```python
from build123d import *

# Parameters (mm, degrees)
SKETCH1_R               = 10
SKETCH1_R_2             = 6.1
BOSS_EXTRUDE1_DEPTH     = 20
SKETCH2_R               = 7
SKETCH2_R_2             = 4
BOSS_EXTRUDE2_DEPTH     = 20
CUT_EXTRUDE1_DEPTH      = 31.000000167
CUT_EXTRUDE1_DEPTH_BACK = 31.000000167
SKETCH5_R               = 6.1


# Read off the part's stored shape, not the designer's step: M3 Tapped Hole1
with BuildPart() as part:
    # Sketch1 → Boss-Extrude1 (new, symmetric)
    with BuildSketch(Plane.XY):
        Circle(SKETCH1_R)
        Circle(SKETCH1_R_2, mode=Mode.SUBTRACT)
    extrude(amount=BOSS_EXTRUDE1_DEPTH, both=True)

    # Sketch2 → Boss-Extrude2 (add, symmetric)
    with BuildSketch(Plane(origin=(0, 0, 0), x_dir=(0, 0, -1), z_dir=(1, 0, 0))):
        Circle(SKETCH2_R)
        with Locations(Location((0, 0, 0), (0, 0, 180))):
            Circle(SKETCH2_R_2, mode=Mode.SUBTRACT)
    extrude(amount=BOSS_EXTRUDE2_DEPTH, both=True)

    # M3 Tapped Hole1 outline → M3 Tapped Hole1 (revolve, cut)
    with BuildSketch(Plane(origin=(17, 0, 0), x_dir=(1, 0, 0), z_dir=(0, 0, 1))):
        Polygon((1.525056823, 7.000056823), (0, 7.000056823), (0, 3.799585789), (1.25, 3.799585789), (1.25, 6.725), align=None)
    revolve(axis=Axis((17, 0, 0), (0, 1, 0)), mode=Mode.SUBTRACT)

    # M3 Tapped Hole1 2 outline → M3 Tapped Hole1 2 (revolve, cut)
    with BuildSketch(Plane(origin=(-17, 0, 0), x_dir=(1, 0, 0), z_dir=(0, 0, 1))):
        Polygon((1.525056823, 7.000056823), (0, 7.000056823), (0, 3.799585789), (1.25, 3.799585789), (1.25, 6.725), align=None)
    revolve(axis=Axis((-17, 0, 0), (0, 1, 0)), mode=Mode.SUBTRACT)

    # Sketch5 → Cut-Extrude1 (cut, two sides: drawn at the far end of the back side and taken through both)
    with BuildSketch(Plane.XY.offset(-CUT_EXTRUDE1_DEPTH_BACK)):
        Circle(SKETCH5_R)
    extrude(amount=CUT_EXTRUDE1_DEPTH + CUT_EXTRUDE1_DEPTH_BACK, mode=Mode.SUBTRACT)


solid = part.part
```
Input: part model. Units: mm. Frame: model coordinates. A direction names the side the tool comes from. Give positions to 0.01 mm unless a question says otherwise; leave off trailing zeros. Write each loop counter-clockwise with the first axis right and the second up, starting at its lowest first coordinate (ties: lowest second). Pieces come first, ordered by that corner, then holes. Notation, with made-up numbers: (73, 16.5) - (91, 16.5) arc R20 ccw to (91, 52.5) - close; hole circle Ø5 at (-14, 69.5). An arc over 180 degrees is marked (long way). Write item = value, one per line. Start each with the question number.
1. Section query D-D, the plane z = -6. Output: boundary loops of the cut face in (x, y).
2. Section query B-B, the plane z = 0. Count the separate pieces of the cut face and the enclosed holes in it, then the cut area to 3 significant figures.
3. Mould query, pull axis Z, two halves, no side actions, for faces 1 (the cylindrical face through (10, 0, 0)), 2 (the cylindrical face through (18.155, 5.283, 0.479)), 3 (the flat face through (-20, -3, -3)), 4 (the cylindrical face through (-13.481, -6.834, 1.517)). Classes: released by +Z, released by -Z, zero draft, split by the parting line, or undercut.
4. Access query for faces 5 (the cylindrical face through (-15.845, 5.283, 0.479)), 6 (the cylindrical face through (-2.17, -9.76, 0.28)), 7 (the cylindrical face through (14.507, -3.966, -0.521)), 8 (the cylindrical face through (-14.66, -2.7, -2.95)). Directions: +Z, -Z, +X, -X, +Y, -Y. A direction counts if a zero-diameter tool reaches every point of the face in a straight line with its end or side. Return the directions, or none.
5. Ray query, L1, parallel to X at y = 0, z = 12.75; L2, parallel to Y at x = -2, z = 10. Return the intervals inside material, ascending.
6. Section query A-A, the plane x = 0. Output: boundary loops of the cut face in (y, z).
7. Section query C-C, the plane y = 0. Output: boundary loops of the cut face in (x, z), then the cut area to 3 significant figures.
8. First-contact query: pin 1 Ø1.5 at (x, z) = (-4, -14) entering from -Y; pin 2 Ø8 at (y, z) = (0.5, 9.5) entering from -X; pin 3 Ø12 at (x, z) = (-7.5, 11) entering from +Y; pin 4 Ø4 at (y, z) = (5.5, 11.5) entering from +X. Flat tips, straight axial feed; report the tip coordinate or a pass-through.
Check sheet entries:
q1.outline = (-20, -3.61) - (-9.33, -3.61) arc R10 ccw to (9.33, -3.61) - (20, -3.61) - (20, 3.61) - (9.33, 3.61) arc R10 ccw to (-9.33, 3.61) - (-20, 3.61) - close; hole circle Ø12.2 at (0, 0)
q2.separate_pieces = 3
q2.enclosed_holes = 1
q2.area = 323 mm2
q3.face_1 = undercut
q3.face_2 = undercut
q3.face_3 = zero draft
q3.face_4 = split by the parting line
q4.face_5 = +Y
q4.face_6 = none
q4.face_7 = +X
q4.face_8 = -X
q5.L1 = -10 to -6.1, 6.1 to 10
q5.L2 = -9.8 to -5.76, 5.76 to 9.8
q6.outline = (-10, -20) - (-6.1, -20) - (-6.1, 20) - (-10, 20) - close; (6.1, -20) - (10, -20) - (10, 20) - (6.1, 20) - close
q7.outline = (-20, -7) - (-10, -7) - (-10, -20) - (-6.1, -20) - (-6.1, 20) - (-10, 20) - (-10, 7) - (-20, 7) - (-20, 4) - (-10, 4) - (-10, -4) - (-20, -4) - close; (6.1, -20) - (10, -20) - (10, -7) - (20, -7) - (20, -4) - (10, -4) - (10, 4) - (20, 4) - (20, 7) - (10, 7) - (10, 20) - (6.1, 20) - close
q7.area = 432 mm2
q8.pin_1 = -9.46
q8.pin_2 = -20
q8.pin_3 = 9.89
q8.pin_4 = 9.37
